Here's how the part is built. I have some questions about the finished solid (model axes, mm). A direction names the side the tool comes from. Coordinates: 2 decimals unless noted, no trailing zeros. Write each loop counter-clockwise with the first axis right and the second up, starting at its lowest first coordinate (ties: lowest second). Pieces come first, ordered by that corner, then holes. Notation, with made-up numbers: (43, 3) -> (63, 3) arc R20 cw to (63, 18) -> close; hole circle Ø9 at (10, 16.25). An arc over 180 degrees is marked (long way). Use a Markdown table: item, result. Add a question column.
Item 1: If I drill on line 1 along Y through (x, z) = (39, 53.5); line 2 along Y through (x, z) = (-33, 72.5); line 3 along Y through (x, z) = (-30, 76), over which ranges is the centre line in solid material (lowest first)? Write a range as from..to.
Item 2: Will these pins go through, and if not, where does the flat tip stop? pin 1 Ø3 at (x, z) = (-30, 53.5) entering from -Y; pin 2 Ø1 at (x, y) = (20.5, 17.5) entering from +Z.
Item 3: Imagine slicing it at C-C, the plane y = -17.5. Write out the boundary of the cut face in (x, z).
Item 4: Imagine slicing it at A-A, the plane z = 40.5. Write out the boundary of the cut face in (x, y), and give its area (3 significant figures).
Item 5: On a 3-axis mill with a long thin cutter (end or side, diameter ignored), from which of +Z, -Z, +X, -X, +Y, -Y can I reach the whole of each face in a straight line? I mean faces 1 (the cylindrical face through (11.421, -90.484, 56.876)), 2 (the cylindrical face through (11.727, -30.504, 70.717)), 3 (the cylindrical face through (12.812, 31.544, 58.062)), 4 (the flat face through (-38, -24, 38.1)). Say none if no direction works.
Item 6: If we mould it in two halves opening along X, with no side actions, what happens to faces 5 (the flat face through (-53.305, -30, 44)), 6 (the cylindrical face through (-46.05, -16.98, 63.86)), 7 (the flat face through (12, -103.361, 70))? For each: pulls with the +X half, pulls with the -X half, needs draft (parallel to the pull), parting line crosses it, or undercut.
Item 7: Imagine slicing it at B-B, the plane x = 63. Write out the boundary of the cut face in (y, z), and give its area (3 significant figures).
Item 8: Imagine slicing it at D-D, the plane x = 6. Write out the boundary of the cut face in (y, z), and give its area (3 significant figures).
```python
from build123d import *

# Parameters (mm, degrees)
F0_W     = 130.8771371841
F0_H     = 96.983704716
F1_DEPTH = 88.9
F3_DEPTH = 25.4
F5_DEPTH = 25.4
F6_R     = 18.1870915774
F7_DEPTH = 147.784704716
F8_R     = 10.7412616006
F8_R_2   = 10.8772665054
F9_DEPTH = 50.8


with BuildPart() as f1:
    # F0 (on Top) → F1 (new body)
    with BuildSketch(Plane.XY):
        with Locations((12.1337100863, -29.4696222991)):
            Rectangle(F0_W, F0_H)
    extrude(amount=F1_DEPTH)

    # F2 (on face) → F3 (join)
    with BuildSketch(Plane(origin=(0, 19.0222300589, 0), x_dir=(-1, 0, 0), z_dir=(0, 1, 0))):
        with BuildLine():
            Line((18.7113173306, 88.9), (-42.9787375033, 88.9))
            ThreePointArc((-42.9787375033, 88.9), (-12.1337100863, 58.0549725831), (18.7113173306, 88.9))
        make_face()
    extrude(amount=F3_DEPTH)

    # F4 (on face) → F5 (join)
    with BuildSketch(Plane.XZ.offset(77.9614746571)):
        with BuildLine():
            Line((44.4338358939, 88.9), (-20.1796386391, 88.9))
            ThreePointArc((-20.1796386391, 88.9), (12.1270986274, 56.8678088056), (44.4338358939, 88.9))
        make_face()
    extrude(amount=F5_DEPTH)

    # F6 (on face) → F7 (cut, through all)
    with BuildSketch(Plane.XZ.offset(103.3614746571)):
        with Locations((12.1270986274, 88.9)):
            Circle(F6_R)
    extrude(amount=-F7_DEPTH, mode=Mode.SUBTRACT)

    # F8 (on face) → F9 (cut)
    with BuildSketch(Plane.XY.offset(88.9)):
        with Locations((60.6468096375, -24.3307966739)):
            Circle(F8_R)
        with Locations((-38.0332432687, -24.3307966739)):
            Circle(F8_R_2)
    extrude(amount=-F9_DEPTH, mode=Mode.SUBTRACT)


solid = f1.part
```
Ans:
| question | item | result |
|---|---|---|
| 1 | line 1 | y = -77.96..19.02 |
| 1 | line 2 | y = -77.96..-33.97, -14.69..19.02 |
| 1 | line 3 | y = -77.96..-31.66, -17..19.02 |
| 2 | pin 1 | stops at y = -77.96 |
| 2 | pin 2 | stops at z = 73.02 |
| 3 | outline | (-53.3, 0) -> (77.57, 0) -> (77.57, 88.9) -> (68.94, 88.9) -> (68.94, 38.1) -> (52.36, 38.1) -> (52.36, 88.9) -> (30.31, 88.9) arc R18.19 cw to (-6.06, 88.9) -> (-29.57, 88.9) -> (-29.57, 38.1) -> (-46.5, 38.1) -> (-46.5, 88.9) -> (-53.3, 88.9) -> close |
| 4 | outline | (-53.3, -77.96) -> (77.57, -77.96) -> (77.57, 19.02) -> (-53.3, 19.02) -> close; hole circle Ø21.75 at (-38.03, -24.33); hole circle Ø21.48 at (60.65, -24.33) |
| 4 | area | 12,000 mm^2 |
| 5 | face 1 | -Z, -Y |
| 5 | face 2 | +Z, +Y, -Y |
| 5 | face 3 | -Z, +Y |
| 5 | face 4 | +Z |
| 6 | face 5 | pulls with the -X half |
| 6 | face 6 | undercut |
| 6 | face 7 | needs draft |
| 7 | outline | (-77.96, 0) -> (19.02, 0) -> (19.02, 88.9) -> (-13.85, 88.9) -> (-13.85, 38.1) -> (-34.81, 38.1) -> (-34.81, 88.9) -> (-77.96, 88.9) -> close |
| 7 | area | 7,560 mm^2 |
| 8 | outline | (-103.36, 57.45) -> (-77.96, 57.45) -> (-77.96, 0) -> (19.02, 0) -> (19.02, 58.67) -> (44.42, 58.67) -> (44.42, 71.78) -> (-103.36, 71.78) -> close |
| 8 | area | 7,660 mm^2 |
